```python
from build123d import *

# Parameters (mm, degrees)
SKETCH1_R           = 57.5
SKETCH1_R_2         = 1.6
BOSS_EXTRUDE1_DEPTH = 10.6
FILLET1_R           = 14


with BuildPart() as part:
    # Sketch1 → Boss-Extrude1 (new body)
    with BuildSketch(Plane(origin=(0, 0, 0), x_dir=(1, 0, 0), z_dir=(0, 1, 0))):
        with Locations(Location((0, 0, 0), (0, 0, 270))):
            Circle(SKETCH1_R)
        with Locations(Location((-27, -46.765371804, 0), (0, 0, 270))):
            Circle(SKETCH1_R_2, mode=Mode.SUBTRACT)
        with Locations(Location((-46.765371804, -27, 0), (0, 0, 270))):
            Circle(SKETCH1_R_2, mode=Mode.SUBTRACT)
        with Locations(Location((-54, 0, 0), (0, 0, 270))):
            Circle(SKETCH1_R_2, mode=Mode.SUBTRACT)
        with Locations(Location((0, -54, 0), (0, 0, 270))):
            Circle(SKETCH1_R_2, mode=Mode.SUBTRACT)
        with Locations(Location((27, -46.765371804, 0), (0, 0, 270))):
            Circle(SKETCH1_R_2, mode=Mode.SUBTRACT)
        with Locations(Location((46.765371804, -27, 0), (0, 0, 270))):
            Circle(SKETCH1_R_2, mode=Mode.SUBTRACT)
        with Locations(Location((-46.765371804, 27, 0), (0, 0, 270))):
            Circle(SKETCH1_R_2, mode=Mode.SUBTRACT)
        with Locations(Location((-27, 46.765371804, 0), (0, 0, 270))):
            Circle(SKETCH1_R_2, mode=Mode.SUBTRACT)
        with BuildLine():
            ThreePointArc((43.337291938, 12.119369929), (44.541964885, 6.404167722), (44.996248187, 0.581075772))
            ThreePointArc((44.996248187, 0.581075772), (49.649801174, -1.617727663), (51.541964885, -6.404167722))
            ThreePointArc((51.541964885, -6.404167722), (48.916629323, -11.868809619), (43.009876012, -13.234446171))
            ThreePointArc((43.009876012, -13.234446171), (40.933439791, -18.693675585), (38.167406032, -23.837976356))
            ThreePointArc((38.167406032, -23.837976356), (40.258159872, -26.3152212), (41.008730846, -29.468733028))
            ThreePointArc((41.008730846, -29.468733028), (36.666623102, -35.944503928), (29.027128345, -34.386419122))
            ThreePointArc((29.027128345, -34.386419122), (24.328836786, -37.856408977), (19.22068214, -40.688639423))
            ThreePointArc((19.22068214, -40.688639423), (19.562695248, -41.91207899), (19.677965058, -43.177183813))
            ThreePointArc((19.677965058, -43.177183813), (13.403758509, -50.139455271), (5.828472525, -44.620946965))
            ThreePointArc((5.828472525, -44.620946965), (0, -45), (-5.828472525, -44.620946965))
            ThreePointArc((-5.828472525, -44.620946965), (-14.650092956, -49.893634628), (-19.22068214, -40.688639423))
            ThreePointArc((-19.22068214, -40.688639423), (-24.328836785, -37.856408977), (-29.027128345, -34.386419122))
            ThreePointArc((-29.027128345, -34.386419122), (-39.298977866, -34.052758165), (-38.167406032, -23.837976356))
            ThreePointArc((-38.167406032, -23.837976356), (-40.933439791, -18.693675585), (-43.009876012, -13.234446171))
            ThreePointArc((-43.009876012, -13.234446171), (-51.470714978, -7.40037159), (-44.996248187, 0.581075772))
            ThreePointArc((-44.996248187, 0.581075772), (-44.541964885, 6.404167722), (-43.337291938, 12.119369929))
            ThreePointArc((-43.337291938, 12.119369929), (-47.300863758, 21.601580676), (-37.539099471, 24.815640449))
            ThreePointArc((-37.539099471, 24.815640449), (-34.008730846, 29.468733028), (-29.905423881, 33.625371708))
            ThreePointArc((-29.905423881, 33.625371708), (-28.113322508, 43.745183707), (-18.163551911, 41.171414622))
            ThreePointArc((-18.163551911, 41.171414622), (-12.677965058, 43.177183813), (-6.978795043, 44.455555556))
            ThreePointArc((-6.978795043, 44.455555556), (-0.272428616, 51.994696752), (7, 45))
            ThreePointArc((7, 45), (6.994696752, 44.727571384), (6.978795043, 44.455555556))
            ThreePointArc((6.978795043, 44.455555556), (12.677965058, 43.177183813), (18.163551911, 41.171414622))
            ThreePointArc((18.163551911, 41.171414622), (26.038077243, 44.644523374), (31.328836786, 37.856408977))
            ThreePointArc((31.328836786, 37.856408977), (30.963447161, 35.624381834), (29.905423881, 33.625371708))
            ThreePointArc((29.905423881, 33.625371708), (34.008730846, 29.468733028), (37.539099471, 24.815640449))
            ThreePointArc((37.539099471, 24.815640449), (44.485876825, 24.725274968), (47.933439791, 18.693675585))
            ThreePointArc((47.933439791, 18.693675585), (46.670467115, 14.68287548), (43.337291938, 12.119369929))
        make_face(mode=Mode.SUBTRACT)
        with Locations(Location((54, 0, 0), (0, 0, 270))):
            Circle(SKETCH1_R_2, mode=Mode.SUBTRACT)
        with Locations(Location((46.765371804, 27, 0), (0, 0, 270))):
            Circle(SKETCH1_R_2, mode=Mode.SUBTRACT)
        with Locations(Location((0, 54, 0), (0, 0, 270))):
            Circle(SKETCH1_R_2, mode=Mode.SUBTRACT)
        with Locations(Location((27, 46.765371804, 0), (0, 0, 270))):
            Circle(SKETCH1_R_2, mode=Mode.SUBTRACT)
    extrude(amount=BOSS_EXTRUDE1_DEPTH)

    # Fillet1
    # the kernel refuses this fillet: 14 mm, written as the material it takes off along each edge
    with BuildSketch(Plane(origin=(43.009876012, -16.77410228, 13.234446171), x_dir=(-0.3645348982341331, 0, 0.9311897271605987), z_dir=(0, 1, 0)), Plane(origin=(43.337291938, -16.77410228, -12.119369929), x_dir=(0.19677290431862063, 0, 0.9804490930823564), z_dir=(0, 1, 0)), Plane(origin=(29.027128345, -16.77410228, 34.386419122), x_dir=(-0.8101054462780665, 0, 0.586284202337582), z_dir=(0, 1, 0)), Plane(origin=(5.828472525, -16.77410228, 44.620946965), x_dir=(-0.9984732390602963, 0, 0.05523758575861507), z_dir=(0, 1, 0)), Plane(origin=(-19.22068214, -16.77410228, 40.688639423), x_dir=(-0.8698328333156817, 0, -0.4933465740085904), z_dir=(0, 1, 0)), Plane(origin=(-38.167406032, -16.77410228, 23.837976356), x_dir=(-0.46502664893844664, 0, -0.8852966823483972), z_dir=(0, 1, 0)), Plane(origin=(-44.996248187, -16.77410228, -0.581075772), x_dir=(0.0874222107554752, 0, -0.99617134925003), z_dir=(0, 1, 0)), Plane(origin=(-37.539099471, -16.77410228, -24.815640449), x_dir=(0.6121151362303556, 0, -0.7907686513751624), z_dir=(0, 1, 0)), Plane(origin=(-18.163551911, -16.77410228, -41.171414622), x_dir=(0.9424658309509625, 0, -0.334302493992958), z_dir=(0, 1, 0)), Plane(origin=(6.978795043, -16.77410228, -44.455555556), x_dir=(0.9735902834899675, 0, 0.22830234316345693), z_dir=(0, 1, 0))) as fillet1_piece_1:
        with BuildLine():
            CenterArc((7.753362832, 13.961040239), FILLET1_R, 225.679308165, 40.045235058)
            ThreePointArc((-2.028069047, 3.944873787), (-0.693306264, 2.137324059), (0, 0))
            ThreePointArc((0, 0), (3.354820456, 0.125227803), (6.709640912, 0))
        make_face()
    extrude(amount=44.14820456, mode=Mode.SUBTRACT)
    with BuildSketch(Plane(origin=(44.996248187, -16.77410228, -0.581075772), x_dir=(0.9259201789863998, 0, 0.37771923719317424), z_dir=(0, 1, 0)), Plane(origin=(37.539099471, -16.77410228, -24.815640449), x_dir=(0.9831440588568181, 0, -0.18283259975874497), z_dir=(0, 1, 0)), Plane(origin=(38.167406032, -16.77410228, 23.837976356), x_dir=(0.5747231845271455, 0, 0.8183478851729116), z_dir=(0, 1, 0)), Plane(origin=(19.22068214, -16.77410228, 40.688639423), x_dir=(0.041055639780420296, 0, 0.9991568617800813), z_dir=(0, 1, 0)), Plane(origin=(-5.828472525, -16.77410228, 44.620946965), x_dir=(-0.5056467805113274, 0, 0.8627405944770012), z_dir=(0, 1, 0)), Plane(origin=(-29.027128345, -16.77410228, 34.386419122), x_dir=(-0.8918099207200904, 0, 0.4524102842611189), z_dir=(0, 1, 0)), Plane(origin=(-43.009876012, -16.77410228, 13.234446171), x_dir=(-0.994829712327915, 0, -0.10155709462936494), z_dir=(0, 1, 0)), Plane(origin=(-43.337291938, -16.77410228, -12.119369929), x_dir=(-0.7819980994024467, 0, -0.62328081354311), z_dir=(0, 1, 0)), Plane(origin=(-29.905423881, -16.77410228, -33.625371708), x_dir=(-0.3208876152512941, 0, -0.9471172780486783), z_dir=(0, 1, 0)), Plane(origin=(18.163551911, -16.77410228, -41.171414622), x_dir=(0.7282266466043301, 0, -0.6853363781205636), z_dir=(0, 1, 0)), Plane(origin=(-6.978795043, -16.77410228, -44.455555556), x_dir=(0.24210241945853378, 0, -0.9702506987847646), z_dir=(0, 1, 0))) as fillet1_piece_2:
        with BuildLine():
            CenterArc((8.87132307, 13.278738899), FILLET1_R, 211.483261097, 40.045235058)
            ThreePointArc((-3.067775786, 5.967246676), (-1.422516032, 3.040879878), (0, 0))
            ThreePointArc((0, 0), (2.217830767, 0.36063055), (4.435661535, 0))
        make_face()
    extrude(amount=44.14820456, mode=Mode.SUBTRACT)
    with BuildSketch(Plane(origin=(29.905423881, -16.77410228, -33.625371708), x_dir=(0.3208876152513925, 0, -0.9471172780486449), z_dir=(0, 1, 0))) as fillet1_piece_3:
        with BuildLine():
            CenterArc((8.87132307, -13.278738899), FILLET1_R, 108.471503845, 40.045235058)
            ThreePointArc((-3.067775786, -5.967246676), (-1.422516032, -3.040879878), (0, 0))
            ThreePointArc((0, 0), (2.217830767, -0.36063055), (4.435661535, 0))
        make_face()
    extrude(amount=44.14820456, mode=Mode.SUBTRACT)


solid = part.part
```
CAD build for the part. Positions are in the model's coordinates, mm. Round coordinates to 2 decimals unless told otherwise and drop trailing zeros. Order: outer loops, then holes, each group sorted by start corner. A loop starts at its lowest first (then second) coordinate and runs counter-clockwise, first axis right, second up.
Q1. Slice it at A-A (z = -27). Write the cut outline in (x, y).
Q2. Slice it at D-D (x = -27). Write the cut outline in (y, z), and give its area (3 significant figures).
Q3. Slice it at B-B (x = 54). Write the cut outline in (y, z), and give its area (3 significant figures).
Q4. Drop flat-ended pins along their axis: pin 1 (5 mm diameter, centred on y = 5, z = 13, fed in from -X); pin 2 (6 mm diameter, centred on x = 19.5, y = 7, fed in from +Z); pin 3 (3 mm diameter, centred on y = 5.5, z = 11.5, fed in from -X). Give the stop position or say it passes through.
Q5. Two-plate mould, pull along Z, no slides. Class faces 1 (the cylindrical face through (0, 5, -52)), 2 (the flat face through (-25, 0, 38)): pulls with the +Z half, pulls with the -Z half, needs draft (parallel to the pull), parting line crosses it, or undercut.
Q6. Wall check: L1, parallel to X at y = 6.5, z = 0; L2, parallel to Z at x = -48, y = 1.5; L3, parallel to Z at x = -12.5, y = 5.75. Give the ranges that are in metal, low to high.
Q7. Slice it at C-C (z = -54). Write the cut outline in (x, y), and give its area (3 significant figures).
Results below:
1. outline: (-50.77, 0) - (-48.37, 0) - (-48.37, 10.6) - (-50.77, 10.6) - close; (-45.17, 0) - (-37.51, 0) - (-37.51, 10.6) - (-45.17, 10.6) - close; (37.51, 0) - (45.17, 0) - (45.17, 10.6) - (37.51, 10.6) - close; (48.37, 0) - (50.77, 0) - (50.77, 10.6) - (48.37, 10.6) - close
2. outline: (0, -50.77) - (10.6, -50.77) - (10.6, -48.37) - (0, -48.37) - close; (0, -45.17) - (10.6, -45.17) - (10.6, -44.33) - (0, -44.33) - close; (0, 36.81) - (10.6, 36.81) - (10.6, 45.17) - (0, 45.17) - close; (0, 48.37) - (10.6, 48.37) - (10.6, 50.77) - (0, 50.77) - close
2. area: 148 mm2
3. outline: (0, -19.75) - (10.6, -19.75) - (10.6, -1.6) - (0, -1.6) - close; (0, 1.6) - (10.6, 1.6) - (10.6, 19.75) - (0, 19.75) - close
3. area: 385 mm2
4. pin 1: stops at x = -56.53
4. pin 2: stops at z = 55.08
4. pin 3: stops at x = -56.62
5. face 1: undercut
5. face 2: needs draft
6. L1: x = -57.5 to -55.6, -52.4 to -47.97, 47.97 to 52.4, 55.6 to 57.5
6. L2: z = -31.66 to -28.02, -25.98 to 0.04, 12.49 to 25.98, 28.02 to 31.66
6. L3: z = -56.12 to -43.29, 50.17 to 56.12
7. outline: (-19.75, 0) - (-1.6, 0) - (-1.6, 10.6) - (-19.75, 10.6) - close; (1.6, 0) - (19.75, 0) - (19.75, 10.6) - (1.6, 10.6) - close
7. area: 385 mm2
